Geometry: see drawing. Coordinates: mm, zero at the bounding-box minimum. A direction names the side the tool comes from. Give positions to 0.01 mm unless a question says otherwise; leave off trailing zeros. Write each loop counter-clockwise with the first axis right and the second up, starting at its lowest first coordinate (ties: lowest second). Pieces come first, ordered by that corner, then holes. Notation, with made-up numbers: (-12.5, 71) - (-3.5, 71) arc R27 ccw to (-3.5, 105) - close; hole circle Ø2 at (66.5, 42). An arc over 180 degrees is marked (long way). Use a Markdown table: item, result. Add a question column.
1. Material intervals for probe 1 along Y at (x, z) = (10, 18); probe 2 along X at (y, z) = (27.5, 35); probe 3 along Z at (x, y) = (7, 17), sorted ascending.
2. Pin query (flat end, axial travel): pin 1 (12 mm diameter, centred on x = 39.5, y = 22.5, fed in from +Z); pin 2 (11.5 mm diameter, centred on y = 29, z = 29.5, fed in from -X); pin 3 (22 mm diameter, centred on x = 34.5, y = 26.5, fed in from -Z); pin 4 (8 mm diameter, centred on x = 51, z = 33, fed in from +Y). Return the tip coordinate at first contact, or that it passes through.
3. Section query D-D, the plane z = 17. Return loops of the section in (x, y).
4. Section query B-B, the plane x = 10. Return loops of the section in (y, z).
5. Mould query, pull axis X, two halves, no side actions, for the marked faces 1, 2 and 3. Classes: released by +X, released by -X, zero draft, split by the parting line, or undercut.
6. Section query A-A, the plane z = 5. Return loops of the section in (x, y).
7. Set-up query: the marked faces 4, 5 and 6. Return all of +Z, -Z, +X, -X, +Y, -Y with unobstructed straight access to the full face (end or side cutting, diameter ignored); none if empty.
8. Section query C-C, the plane y = 20. Return loops of the section in (x, z) (1 decimal).
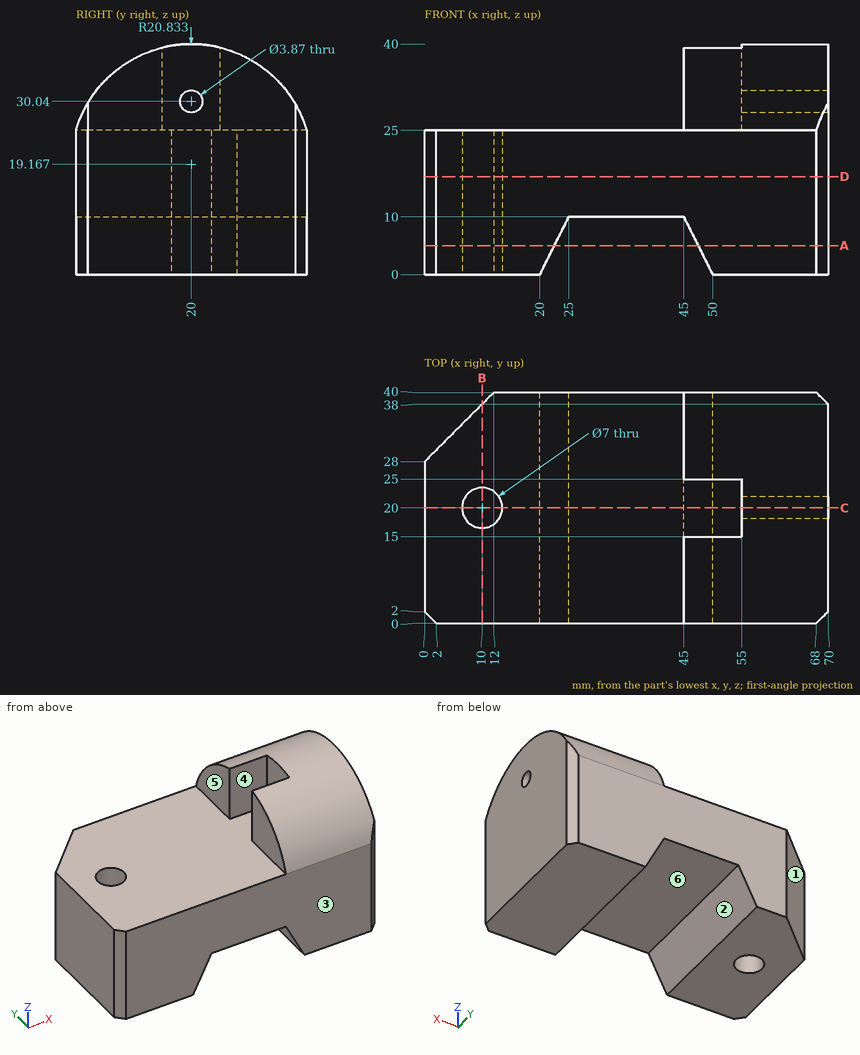
Result sheet:
| question | item | result |
|---|---|---|
| 1 | probe 1 | y = 0 to 16.5, 23.5 to 38 |
| 1 | probe 2 | x = 45 to 70 |
| 1 | probe 3 | z = 0 to 25 |
| 2 | pin 1 | stops at z = 25 |
| 2 | pin 2 | stops at x = 0 |
| 2 | pin 3 | stops at z = 7 |
| 2 | pin 4 | stops at y = 38.37 |
| 3 | outline | (0, 2) - (2, 0) - (68, 0) - (70, 2) - (70, 38) - (68, 40) - (12, 40) - (0, 28) - close; hole circle Ø7 at (10, 20) |
| 4 | outline | (0, 0) - (16.5, 0) - (16.5, 25) - (0, 25) - close; (23.5, 0) - (38, 0) - (38, 25) - (23.5, 25) - close |
| 5 | face 1 | released by -X |
| 5 | face 2 | undercut |
| 5 | face 3 | zero draft |
| 6 | outline | (0, 2) - (2, 0) - (22.5, 0) - (22.5, 40) - (12, 40) - (0, 28) - close; (47.5, 0) - (68, 0) - (70, 2) - (70, 38) - (68, 40) - (47.5, 40) - close; hole circle Ø7 at (10, 20) |
| 7 | face 4 | +Z, -X |
| 7 | face 5 | +Z, -X, +Y, -Y |
| 7 | face 6 | -Z, +Y, -Y |
| 8 | outline | (0, 0) - (6.5, 0) - (6.5, 25) - (0, 25) - close; (13.5, 0) - (20, 0) - (25, 10) - (45, 10) - (50, 0) - (70, 0) - (70, 28.1) - (55, 28.1) - (55, 25) - (13.5, 25) - close; (55, 32) - (70, 32) - (70, 40) - (55, 40) - close |
